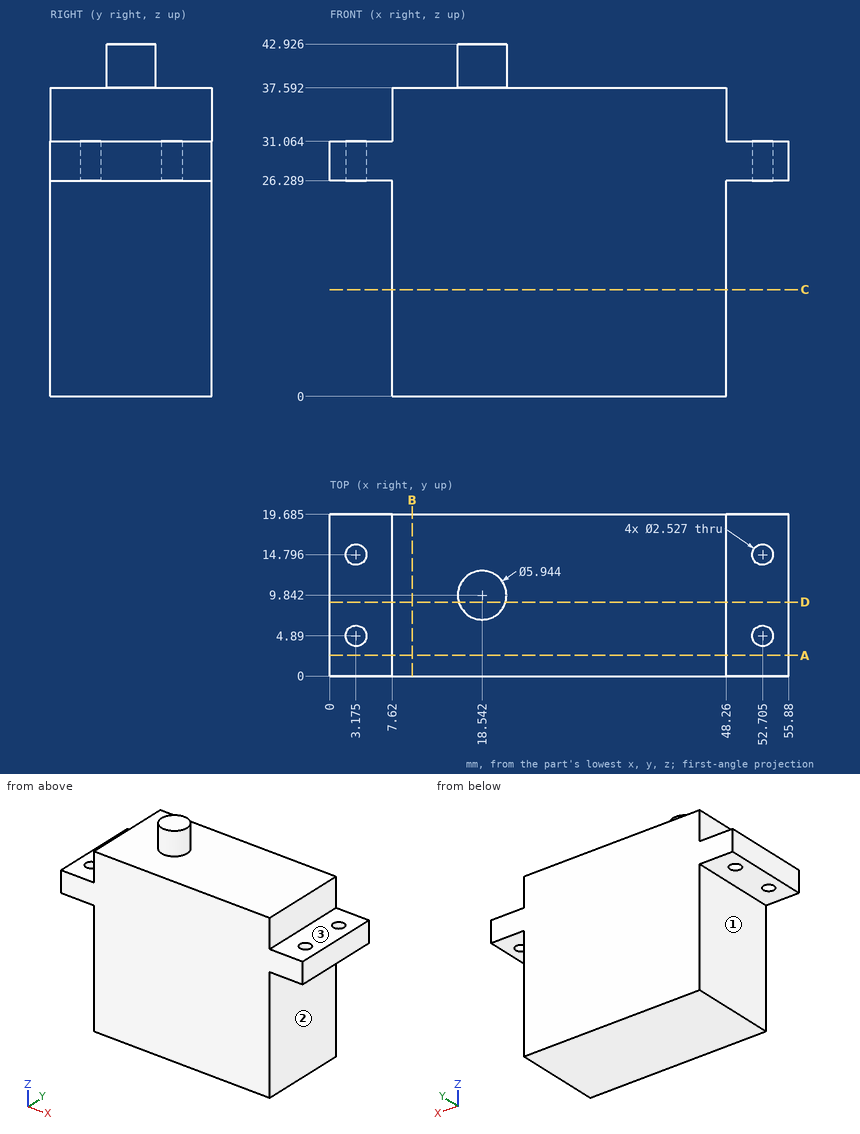
Could you check a few things on this drawing? It's one solid part, dimensions in mm from its lowest x, y, z. A direction names the side the tool comes from. Coordinates: 2 decimals unless noted, no trailing zeros. Order: outer loops, then holes, each group sorted by start corner. A loop starts at its lowest first (then second) coordinate and runs counter-clockwise, first axis right, second up. Notation, with made-up numbers: M 54,84 L 86,84 A8 ccw 86,93 Z; hole C -35,5.5 d5. An arc over 180 degrees is marked long. Answer as a JSON object with one key per item and string values. Group by question number.
(1) Suppose I cut it at A-A, the plane y = 2.5. Please give me the cut outline in (x, z) (1 decimal).
(2) Suppose I cut it at C-C, the plane z = 13. Please give me the cut outline in (x, y) (1 decimal), then the cut area to 3 significant figures.
(3) I need wall thicknesses on probe 1 along Z at (x, y) = (34.5, 17.5); probe 2 along X at (y, z) = (6.25, 14.5); probe 3 along Y at (x, z) = (52.5, 27.5) (1 decimal). Which ranges of each line are inside material? Lowest first, please.
(4) For pin 1 (3 mm diameter, centred on x = 26, z = 17, fed in from -Y); pin 2 (4 mm diameter, centred on x = 3.17, y = 4.89, fed in from +Z); pin 3 (2.5 mm diameter, centred on x = 52, y = 7.5, fed in from -Z); pin 4 (6 mm diameter, centred on x = 8.5, y = 14, fed in from +Z), each with a flat end and sliding along its axis, tell me the tip position at first contact or that it passes through.
(5) Suppose I cut it at B-B, the plane x = 10. Please give me the cut outline in (y, z) (1 decimal), then the cut area to 3 significant figures.
(6) Suppose I cut it at D-D, the plane y = 9. Please give me the cut outline in (x, z) (1 decimal), then the cut area to 3 significant figures.
(7) Which directions (+Z, -Z, +X, -X, +Y, -Y) give clear straight access to the entire face, cutting with the end or side of a thin tool? Please do the marked faces 1, 2 and 3.
Values found:
{
 "1": {"outline": "M 0,26.3 L 7.6,26.3 L 7.6,0 L 48.3,0 L 48.3,26.3 L 55.9,26.3 L 55.9,31.1 L 48.3,31.1 L 48.3,37.6 L 7.6,37.6 L 7.6,31.1 L 0,31.1 Z"},
 "2": {"outline": "M 7.6,0 L 48.3,0 L 48.3,19.7 L 7.6,19.7 Z", "area": "800 mm^2"},
 "3": {"probe 1": "z = 0 to 37.59", "probe 2": "x = 7.62 to 48.26", "probe 3": "y = 0 to 3.6, 6.1 to 13.5, 16 to 19.7"},
 "4": {"pin 1": "stops at y = 0", "pin 2": "stops at z = 31.06", "pin 3": "stops at z = 26.29", "pin 4": "stops at z = 37.59"},
 "5": {"outline": "M 0,0 L 19.7,0 L 19.7,37.6 L 0,37.6 Z", "area": "740 mm^2"},
 "6": {"outline": "M 0,26.3 L 7.6,26.3 L 7.6,0 L 48.3,0 L 48.3,26.3 L 55.9,26.3 L 55.9,31.1 L 48.3,31.1 L 48.3,37.6 L 21.4,37.6 L 21.4,42.9 L 15.7,42.9 L 15.7,37.6 L 7.6,37.6 L 7.6,31.1 L 0,31.1 Z", "area": "1,630 mm^2"},
 "7": {"face 1": "-Z, -X, +Y, -Y", "face 2": "-Z, +X, +Y, -Y", "face 3": "+Z, +X, +Y, -Y"}
}
